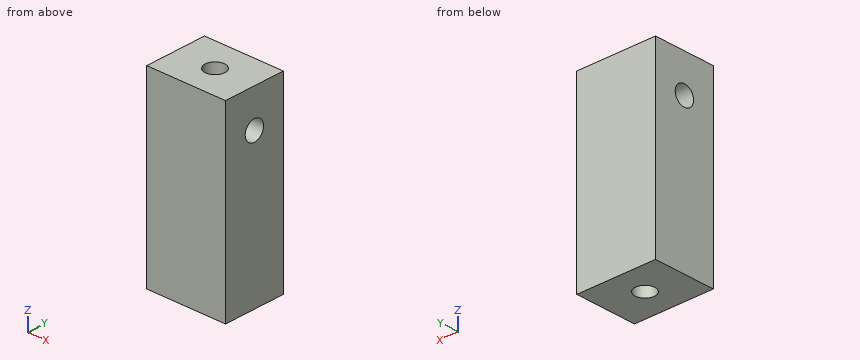
from build123d import *

# Parameters (mm, degrees)
SKETCH1_W           = 12.7
SKETCH1_H           = 10
SKETCH1_R           = 1.5875
BOSS_EXTRUDE1_DEPTH = 30
SKETCH2_R           = 1.59
CUT_EXTRUDE1_DEPTH  = 30


with BuildPart() as part:
    # Sketch1 → Boss-Extrude1 (new body)
    with BuildSketch(Plane.XY):
        with Locations((6.35, -5)):
            Rectangle(SKETCH1_W, SKETCH1_H)
        with Locations((6.35, -5)):
            Circle(SKETCH1_R, mode=Mode.SUBTRACT)
    extrude(amount=BOSS_EXTRUDE1_DEPTH)

    # Sketch2 → Cut-Extrude1 (cut)
    with BuildSketch(Plane(origin=(0, 0, 0), x_dir=(0, 0, -1), z_dir=(1, 0, 0))):
        with Locations((-24, -5)):
            Circle(SKETCH2_R)
    extrude(amount=CUT_EXTRUDE1_DEPTH, mode=Mode.SUBTRACT)


solid = part.part
Check sheet for the modelled part. Datum: model origin and axes. Units: mm. Coordinates: 2 decimals unless noted, no trailing zeros. Write each loop counter-clockwise with the first axis right and the second up, starting at its lowest first coordinate (ties: lowest second). Pieces come first, ordered by that corner, then holes.
Item 1: Scan lines: probe 1 along Y at (x, z) = (6.35, 9); probe 2 along X at (y, z) = (-5, 25.85); probe 3 along Z at (x, y) = (1.5, -5.25). Record each from-to range of solid material in increasing order.
Numbers:
probe 1: y = -10 to -6.59, -3.41 to 0
probe 2: x = 0 to 4.76, 7.94 to 12.7
probe 3: z = 0 to 22.43, 25.57 to 30
Item 2: Cross-section at A-A on x = 6.35. Record the boundary of the cut face in (y, z).
Numbers:
outline: (-10, 0) - (-6.59, 0) - (-6.59, 23.91) arc R1.59 cw to (-6.59, 24.09) - (-6.59, 30) - (-10, 30) - close; (-3.41, 0) - (0, 0) - (0, 30) - (-3.41, 30) - (-3.41, 24.09) arc R1.59 cw to (-3.41, 23.91) - close
Item 3: Cross-section at D-D on x = 9.75. Record the boundary of the cut face in (y, z), then the cut area to 3 significant figures.
Numbers:
outline: (-10, 0) - (0, 0) - (0, 30) - (-10, 30) - close; hole circle Ø3.18 at (-5, 24)
area: 292 mm2
Item 4: Cross-section at B-B on y = -5.75. Record the boundary of the cut face in (x, z), then the cut area to 3 significant figures.
Numbers:
outline: (0, 0) - (4.95, 0) - (4.95, 22.6) - (0, 22.6) - close; (0, 25.4) - (4.95, 25.4) - (4.95, 30) - (0, 30) - close; (7.75, 0) - (12.7, 0) - (12.7, 22.6) - (7.75, 22.6) - close; (7.75, 25.4) - (12.7, 25.4) - (12.7, 30) - (7.75, 30) - close
area: 269 mm2
